```python
from build123d import *

# Parameters (mm, degrees)
SKETCH1_W           = 60
SKETCH1_H           = 20
BOSS_EXTRUDE2_DEPTH = 12.7
FILLET1_R           = 2.54
FILLET2_R           = 2.54
SKETCH2_R           = 5
BOSS_EXTRUDE3_DEPTH = 25.4


with BuildPart() as part:
    # Sketch1 → Boss-Extrude2 (new body)
    with BuildSketch(Plane.XY):
        with Locations((-52.498731257, -25.490525622)):
            Rectangle(SKETCH1_W, SKETCH1_H)
    extrude(amount=BOSS_EXTRUDE2_DEPTH)

    # Fillet1
    fillet1_edges = [part.edges().sort_by_distance(p)[0] for p in [
        (-52.498731257, -35.490525622, 0),
    ]]
    fillet(fillet1_edges, radius=FILLET1_R)

    # Fillet2
    fillet2_edges = [part.edges().sort_by_distance(p)[0] for p in [
        (-52.498731257, -15.490525622, 0),
    ]]
    fillet(fillet2_edges, radius=FILLET2_R)

    # Sketch2 → Boss-Extrude3 (add)
    with BuildSketch(Plane(origin=(0, 0, 0), x_dir=(-1, 0, 0), z_dir=(0, 0, -1))):
        with Locations((74.89901914, -24.866644028)):
            Circle(SKETCH2_R)
    extrude(amount=BOSS_EXTRUDE3_DEPTH)


solid = part.part
```
Check sheet for the modelled part. Datum: model origin and axes. Units: mm. A direction names the side the tool comes from. Give positions to 0.01 mm unless a question says otherwise; leave off trailing zeros. Loops run counter-clockwise (first coordinate to the right, second up) from the corner with the lowest first, then second, coordinate; pieces in that order, holes last. Notation, with made-up numbers: (-17.5, 85.25) - (13.5, 85.25) arc R25 cw to (13.5, 122.25) - close; hole circle Ø9 at (70.25, 8.25). An arc over 180 degrees is marked (long way). One line per question, with ' | ' between items. Start each with the question number.
1. Cross-section at A-A, the plane x = -38.5. Enter the section's corners in (y, z).
2. Set-up check for faces 1 (the cylindrical face through (-71.2, -21.5, -12.5)), 2 (the flat face through (-75, -25, -25.4)): record each of +Z, -Z, +X, -X, +Y, -Y from which the full face is reachable in a straight line by a thin tool's end or side.
3. Cross-section at B-B, the plane y = -23. Enter the section's corners in (x, z).
4. Cross-section at D-D, the plane y = -26.5. Enter the section's corners in (x, z).
5. Gauge pin test, flat ends, axial feed: pin 1 Ø7.5 at (x, y) = (-41.5, -29) entering from -Z; pin 2 Ø8 at (x, z) = (-69, -3.5) entering from -Y; pin 3 Ø10 at (y, z) = (-29, -9) entering from -X. Record the tip position at first contact, or that the pin passes through.
6. Material ranges on line 1 along Z through (x, y) = (-68, -30.75); line 2 along X through (y, z) = (-29.25, -1.5); line 3 along Y through (x, z) = (-74, -21), recorded low to high. Write a range as [from, to].
7. Cross-section at C-C, the plane z = -16.5. Enter the section's corners in (x, y), plus the area to 3 significant figures.
Check result:
1) outline: (-35.49, 2.54) arc R2.54 ccw to (-32.95, 0) - (-18.03, 0) arc R2.54 ccw to (-15.49, 2.54) - (-15.49, 12.7) - (-35.49, 12.7) - close
2) face 1: -Z | face 2: -Z, +X, -X, +Y, -Y
3) outline: (-82.5, 0) - (-79.54, 0) - (-79.54, -25.4) - (-70.26, -25.4) - (-70.26, 0) - (-22.5, 0) - (-22.5, 12.7) - (-82.5, 12.7) - close
4) outline: (-82.5, 0) - (-79.62, 0) - (-79.62, -25.4) - (-70.17, -25.4) - (-70.17, 0) - (-22.5, 0) - (-22.5, 12.7) - (-82.5, 12.7) - close
5) pin 1: stops at z = 0 | pin 2: stops at y = -34.46 | pin 3: stops at x = -79.9
6) line 1: z = [0, 12.7] | line 2: x = [-77.3, -72.49] | line 3: y = [-29.79, -19.95]
7) outline: circle Ø10 at (-74.9, -24.87) | area: 78.5 mm2
